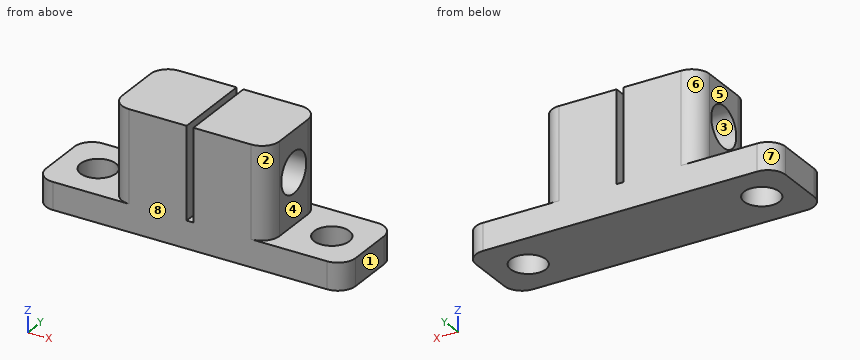
from build123d import *

# Parameters (mm, degrees)
F3_W      = 45.6
F3_H      = 12
F3_R      = 2.6
F4_DEPTH  = 4
F5_W      = 23.2
F5_H      = 12
F6_DEPTH  = 13.5
F7_R      = 3
F8_DEPTH  = 23.2
F9_W      = 1
F9_H      = 12
F10_DEPTH = 13.5
F11_R     = 2.6


with BuildPart() as f4:
    # F3 (on Top) → F4 (new body)
    with BuildSketch(Plane.XY):
        Rectangle(F3_W, F3_H)
        with Locations((-17.2, 0)):
            Circle(F3_R, mode=Mode.SUBTRACT)
        with Locations((17.2, 0)):
            Circle(F3_R, mode=Mode.SUBTRACT)
    extrude(amount=F4_DEPTH)

    # F5 (on face) → F6 (join)
    with BuildSketch(Plane.XY.offset(4)):
        Rectangle(F5_W, F5_H)
    extrude(amount=F6_DEPTH)

    # F7 (on face) → F8 (cut, through all)
    with BuildSketch(Plane.YZ.offset(11.6)):
        with Locations((0, 11.5)):
            Circle(F7_R)
    extrude(amount=-F8_DEPTH, mode=Mode.SUBTRACT)

    # F9 (on face) → F10 (cut, through all)
    with BuildSketch(Plane.XY.offset(17.5)):
        Rectangle(F9_W, F9_H)
    extrude(amount=-F10_DEPTH, mode=Mode.SUBTRACT)

    # F11
    f11_edges = [f4.edges().sort_by_distance(p)[0] for p in [
        (-22.8, -6, 2),
        (-22.8, 6, 2),
        (22.8, -6, 2),
        (22.8, 6, 2),
        (-11.6, 6, 10.75),
        (-11.6, -6, 10.75),
        (11.6, 6, 10.75),
        (11.6, -6, 10.75),
    ]]
    fillet(f11_edges, radius=F11_R)


solid = f4.part
Design review of the part built by this model. Coordinates are the model's own, in mm. Face numbers are marked on the shaded views. A direction names the side the tool comes from. Coordinates: 2 decimals unless noted, no trailing zeros. Write each loop counter-clockwise with the first axis right and the second up, starting at its lowest first coordinate (ties: lowest second). Pieces come first, ordered by that corner, then holes. Notation, with made-up numbers: (22, 35) - (46, 35) arc R8 cw to (46, 47) - close; hole circle Ø11 at (-13, -37). An arc over 180 degrees is marked (long way). Use one line per item in the form item = value.
Q1. For probe 1 along Z at (x, y) = (-7.75, 0); probe 2 along Y at (x, z) = (-17.2, 2.4); probe 3 along X at (y, z) = (2.25, 0.75), list the stretches that pass through material, from the lowest coordinate up.
Taken from the geometry:
probe_1 = 0 to 8.5, 14.5 to 17.5
probe_2 = -6 to -2.6, 2.6 to 6
probe_3 = -22.8 to -18.5, -15.9 to 15.9, 18.5 to 22.8
Q2. Insertion check: pin 1 Ø3 at (x, y) = (16, 1) entering from +Z; pin 2 Ø4 at (x, y) = (-17.2, 0) entering from -Z; pin 3 Ø5.5 at (y, z) = (0, 9) entering from +X; pin 4 Ø2 at (y, z) = (0.5, 7.5) entering from -X. Each pin has a flat end and moves straight along its axis. Give the tip position at first contact, or say it passes through.
Taken from the geometry:
pin_1 = 4
pin_2 = through
pin_3 = 11.6
pin_4 = -11.6
Q3. Consider section C-C (z = 6.5). Write out the cut boundary in (x, y), plus the area to 3 significant figures.
Taken from the geometry:
outline = (-11.6, -3.4) arc R2.6 ccw to (-9, -6) - (-0.5, -6) - (-0.5, 6) - (-9, 6) arc R2.6 ccw to (-11.6, 3.4) - close; (0.5, -6) - (9, -6) arc R2.6 ccw to (11.6, -3.4) - (11.6, 3.4) arc R2.6 ccw to (9, 6) - (0.5, 6) - close
area = 261 mm^2
Q4. Machinability: for the marked faces 4, 5, 6, 7 and 8, which of the approach directions +Z, -Z, +X, -X, +Y, -Y give a long, thin tool a straight path to every point of the face, cutting with its end or side? Answer none if there is none.
Taken from the geometry:
face_4 = +Z, +X, +Y, -Y
face_5 = +Z, -X, +Y, -Y
face_6 = +Z, -X, +Y
face_7 = +Z, -Z, -X, +Y
face_8 = +Z, -Z, +X, -X, -Y
Q5. The part is to be moulded in two halves that separate along Y. For the marked faces 1, 2 and 3, say which applies: +Y half, -Y half, draft (parallel to the pull), parting line (faces both ways), or undercut.
Taken from the geometry:
face_1 = draft
face_2 = -Y half
face_3 = undercut
Q6. Consider section D-D (z = 11.5). Write out the cut boundary in (x, y), plus the area to 3 significant figures.
Taken from the geometry:
outline = (-11.6, -3.4) arc R2.6 ccw to (-9, -6) - (-0.5, -6) - (-0.5, -3) - (-11.6, -3) - close; (-11.6, 3) - (-0.5, 3) - (-0.5, 6) - (-9, 6) arc R2.6 ccw to (-11.6, 3.4) - close; (0.5, -6) - (9, -6) arc R2.6 ccw to (11.6, -3.4) - (11.6, -3) - (0.5, -3) - close; (0.5, 3) - (11.6, 3) - (11.6, 3.4) arc R2.6 ccw to (9, 6) - (0.5, 6) - close
area = 127 mm^2
Q7. Consider section A-A (y = 0). Write out the cut boundary in (x, z).
Taken from the geometry:
outline = (-22.8, 0) - (-19.8, 0) - (-19.8, 4) - (-22.8, 4) - close; (-14.6, 0) - (14.6, 0) - (14.6, 4) - (11.6, 4) - (11.6, 8.5) - (0.5, 8.5) - (0.5, 4) - (-0.5, 4) - (-0.5, 8.5) - (-11.6, 8.5) - (-11.6, 4) - (-14.6, 4) - close; (-11.6, 14.5) - (-0.5, 14.5) - (-0.5, 17.5) - (-11.6, 17.5) - close; (0.5, 14.5) - (11.6, 14.5) - (11.6, 17.5) - (0.5, 17.5) - close; (19.8, 0) - (22.8, 0) - (22.8, 4) - (19.8, 4) - close
Q8. Consider section B-B (x = 17.2). Write out the cut boundary in (y, z), plus the area to 3 significant figures.
Taken from the geometry:
outline = (-6, 0) - (-2.6, 0) - (-2.6, 4) - (-6, 4) - close; (2.6, 0) - (6, 0) - (6, 4) - (2.6, 4) - close
area = 27.2 mm^2
